Check sheet for the drawn part. Datum: minimum x, y, z corner. Units: mm. A direction names the side the tool comes from. Round coordinates to 2 decimals unless told otherwise and drop trailing zeros. Write each loop counter-clockwise with the first axis right and the second up, starting at its lowest first coordinate (ties: lowest second). Pieces come first, ordered by that corner, then holes. Notation, with made-up numbers: M -32.75,-8 L 11.25,-8 A18 cw 11.25,6 Z; hole C -16,3.25 d5. An arc over 180 degrees is marked long. One line per item, written item: value. Start each with the question number.
1. Section check C-C (z = 10). Record the boundary of the cut face in (x, y).
2. Section check A-A (y = 10.75). Record the boundary of the cut face in (x, z).
3. Access from +Z, -Z, +X, -X, +Y, -Y to the whole of each face (thin tool, end or side, straight path). Record for the marked faces 4 and 5.
4. Release check for a two-part mould opening along X. For the marked faces 1, 2 and 3 record: pulls with the +X half, pulls with the -X half, needs draft (parallel to the pull), parting line crosses it, or undercut.
5. Section check B-B (x = 7.5). Record the boundary of the cut face in (y, z).
6. Scan lines: probe 1 along X at (y, z) = (7.25, 38.5); probe 2 along Y at (x, z) = (6, 23.5); probe 3 along X at (y, z) = (13.5, 56.5). Record each from-to range of solid material in increasing order. Write a range as [from, to].
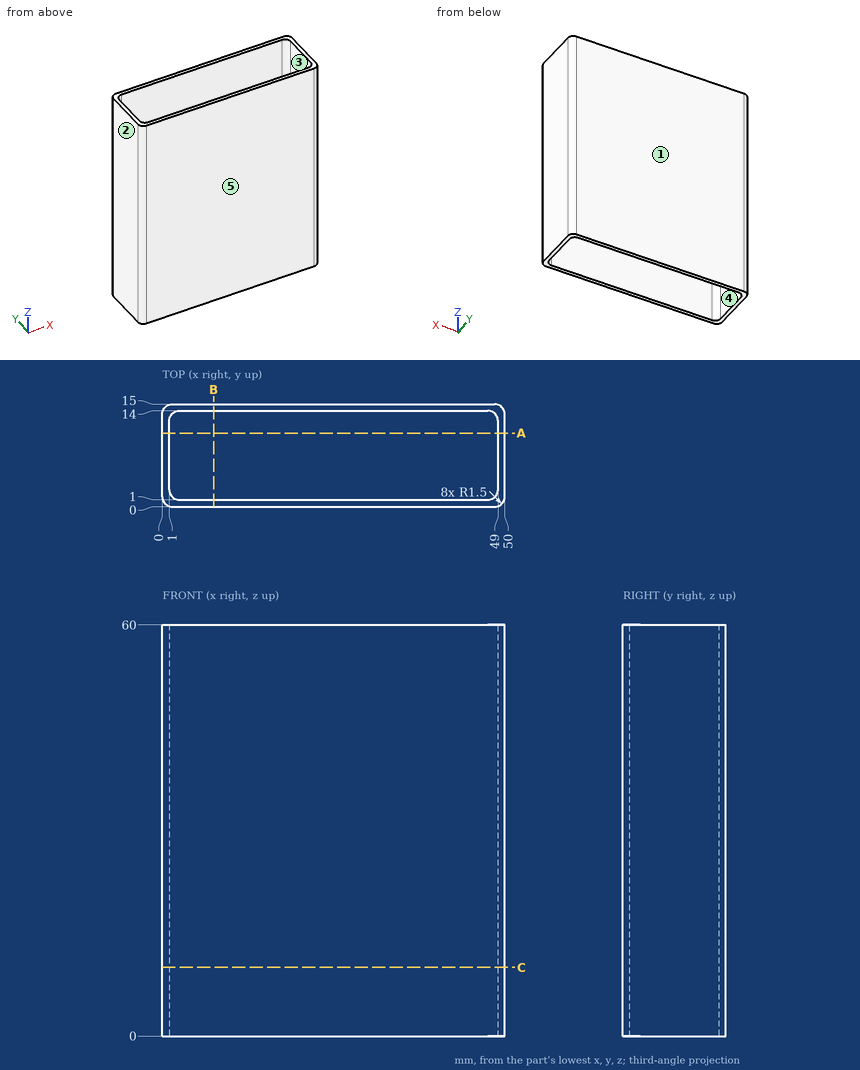
Result sheet:
1. outline: M 0,1.5 A1.5 ccw 1.5,0 L 48.5,0 A1.5 ccw 50,1.5 L 50,13.5 A1.5 ccw 48.5,15 L 1.5,15 A1.5 ccw 0,13.5 Z; hole M 1,2.5 A1.5 ccw 2.5,1 L 47.5,1 A1.5 ccw 49,2.5 L 49,12.5 A1.5 ccw 47.5,14 L 2.5,14 A1.5 ccw 1,12.5 Z
2. outline: M 0,0 L 1,0 L 1,60 L 0,60 Z; M 49,0 L 50,0 L 50,60 L 49,60 Z
3. face 4: +Z, -Z
3. face 5: +Z, -Z, +X, -X, -Y
4. face 1: needs draft
4. face 2: pulls with the -X half
4. face 3: undercut
5. outline: M 0,0 L 1,0 L 1,60 L 0,60 Z; M 14,0 L 15,0 L 15,60 L 14,60 Z
6. probe 1: x = [0, 1], [49, 50]
6. probe 2: y = [0, 1], [14, 15]
6. probe 3: x = [0, 1.38], [48.62, 50]
